from build123d import *

# Parameters (mm, degrees)
F0_W     = 50
F0_H     = 110
F1_DEPTH = 60
F2_W     = 50
F2_H     = 50
F3_DEPTH = 30
F4_W     = 50
F4_H     = 15
F5_DEPTH = 5
F6_W     = 30
F6_H     = 20
F7_DEPTH = 92


with BuildPart() as f1:
    # F0 (on Top) → F1 (new body)
    with BuildSketch(Plane.XY):
        with Locations((3.536819, 18.06074)):
            Rectangle(F0_W, F0_H)
    extrude(amount=F1_DEPTH)

    # F2 (on face) → F3 (cut)
    with BuildSketch(Plane.XY.offset(60)):
        with Locations((3.536819, -11.93926)):
            Rectangle(F2_W, F2_H)
    extrude(amount=-F3_DEPTH, mode=Mode.SUBTRACT)

    # F4 (on face) → F5 (cut)
    with BuildSketch(Plane.XY.offset(30)):
        with Locations((3.536819, -19.43926)):
            Rectangle(F4_W, F4_H)
    extrude(amount=-F5_DEPTH, mode=Mode.SUBTRACT)

    # F6 (on face) → F7 (cut)
    with BuildSketch(Plane(origin=(-21.463181, 0, 0), x_dir=(0, -1, 0), z_dir=(-1, 0, 0))):
        with Locations((-53.06074, 30)):
            Rectangle(F6_W, F6_H)
    extrude(amount=-F7_DEPTH, mode=Mode.SUBTRACT)


solid = f1.part
Input: part model. Units: mm. Frame: model coordinates. A direction names the side the tool comes from. Round coordinates to 2 decimals unless told otherwise and drop trailing zeros. Loops run counter-clockwise (first coordinate to the right, second up) from the corner with the lowest first, then second, coordinate; pieces in that order, holes last. Notation, with made-up numbers: (47.5, -36) -> (51.5, -36) arc R25 ccw to (51.5, -23) -> close; hole circle Ø5 at (-4.75, -36). An arc over 180 degrees is marked (long way). Answer as a JSON object with one key per item and string values. Group by question number.
1) Ray query, L1, parallel to Z at x = -19, y = 52; L2, parallel to Y at x = 3, z = 23; L3, parallel to Y at x = -13, z = 46.5. Return the intervals inside material, ascending.
2) Section query B-B on z = 26.5. Output: boundary loops of the cut face in (x, y), plus the area to 3 significant figures.
3) Pin query (flat end, axial travel): pin 1 (12 mm diameter, centred on x = 0, y = -24, fed in from +Z); pin 2 (24 mm diameter, centred on x = 1.5, z = 50, fed in from -Y). Return the tip coordinate at first contact, or that it passes through.
4) Section query D-D on z = 36.5. Output: boundary loops of the cut face in (x, y).
5) Section query C-C on x = -9.5. Output: boundary loops of the cut face in (y, z), plus the area to 4 significant figures.
6) Section query A-A on y = 66. Output: boundary loops of the cut face in (x, z), plus the area to 3 significant figures.
7) Reachability of faces 4 (the flat face through (3, 1, 30)), 5 (the flat face through (3, 19, 0)), 6 (the flat face through (3, 53, 20)), 7 (the flat face through (3, -19, 25)) from +Z, -Z, +X, -X, +Y, -Y: full face, straight path, thin tool, end or side. Return the list, or none.
8) Draft query along Y for faces 1 (the flat face through (3, 43, 60)), 2 (the flat face through (3, -26.939, 28)), 3 (the flat face through (3, -36.939, 15)). Return one class per face: +Y half, -Y half, draft (parallel to the pull), parting line (faces both ways), or undercut.
Reply:
{
 "1": {"L1": "z = 0 to 20, 40 to 60", "L2": "y = -36.94 to 38.06, 68.06 to 73.06", "L3": "y = 13.06 to 73.06"},
 "2": {"outline": "(-21.46, -36.94) -> (28.54, -36.94) -> (28.54, -26.94) -> (-21.46, -26.94) -> close; (-21.46, -11.94) -> (28.54, -11.94) -> (28.54, 38.06) -> (-21.46, 38.06) -> close; (-21.46, 68.06) -> (28.54, 68.06) -> (28.54, 73.06) -> (-21.46, 73.06) -> close", "area": "3,250 mm2"},
 "3": {"pin 1": "stops at z = 30", "pin 2": "stops at y = 13.06"},
 "4": {"outline": "(-21.46, 13.06) -> (28.54, 13.06) -> (28.54, 38.06) -> (-21.46, 38.06) -> close; (-21.46, 68.06) -> (28.54, 68.06) -> (28.54, 73.06) -> (-21.46, 73.06) -> close"},
 "5": {"outline": "(-36.94, 0) -> (73.06, 0) -> (73.06, 60) -> (13.06, 60) -> (13.06, 30) -> (-11.94, 30) -> (-11.94, 25) -> (-26.94, 25) -> (-26.94, 30) -> (-36.94, 30) -> close; hole (38.06, 20) -> (68.06, 20) -> (68.06, 40) -> (38.06, 40) -> close", "area": "4,425 mm2"},
 "6": {"outline": "(-21.46, 0) -> (28.54, 0) -> (28.54, 20) -> (-21.46, 20) -> close; (-21.46, 40) -> (28.54, 40) -> (28.54, 60) -> (-21.46, 60) -> close", "area": "2,000 mm2"},
 "7": {"face 4": "+Z, +X, -X, -Y", "face 5": "-Z, +X, -X, +Y, -Y", "face 6": "+X, -X", "face 7": "+Z, +X, -X"},
 "8": {"face 1": "draft", "face 2": "undercut", "face 3": "-Y half"}
}
